Source: CAD feature listing. Evaluate the final solid. Frame: model axes, mm. A direction names the side the tool comes from. Round coordinates to 2 decimals unless told otherwise and drop trailing zeros. Loops run counter-clockwise (first coordinate to the right, second up) from the corner with the lowest first, then second, coordinate; pieces in that order, holes last.
Item 1: Section query D-D on y = 2.65. Give the number of separate pieces and of enclosed holes in the cut face, then the cut area to 3 significant figures.
Item 2: First-contact query: P1, Ø4, axis at x = 14, z = 0, coming from the +Y side; P2, Ø5, axis at x = 0, z = -14, coming from the +Y side; P3, Ø2, axis at x = 51.5, y = 1.5, coming from the -Z side; P4, Ø1.2, axis at x = 43, y = 2, coming from the +Z side. Flat tips, straight axial feed; report the tip coordinate or a pass-through.
Item 3: Section query B-B on z = -22.5. Return loops of the section in (x, y).
Item 4: Section query C-C on x = 25. Return loops of the section in (y, z).
Item 5: Pull-direction query (X, two-part tool) for faces 1 (the cylindrical face through (26.16, 1.97, 11.18)), 2 (the flat face through (-28.284, 2, 0)), 3 (the flat face through (41, 2, -15.91)); classes: released by +X, released by -X, zero draft, split by the parting line, or undercut.
Item 6: Access query for faces 4 (the flat face through (41, 2, 15.91)), 5 (the cylindrical face through (0.09, 1.97, 11.9)). Directions: +Z, -Z, +X, -X, +Y, -Y. A direction counts if a zero-diameter tool reaches every point of the face in a straight line with its end or side. Return the directions, or none.
Item 7: Ray query, L1, parallel to X at y = 1.8, z = 0; L2, parallel to Z at x = 59.5, y = 1.1; L3, parallel to Z at x = 50, y = 2.4. Return the intervals inside material, ascending.
Item 8: Section query A-A on x = 0. Return loops of the section in (y, z).
```python
from build123d import *

# Parameters (mm, degrees)
SKETCH_1_R          = 2.1
SKETCH_1_R_2        = 10.5
SKETCH_1_R_3        = 10
EXTRUDE_1_DEPTH     = 4
CHAMFER_1_SIZE      = 5
FILLET_1_R          = 10
SKETCH_2_R          = 2.1
CUT_EXTRUDE_1_DEPTH = 10
EXTRUDE_START       = -3
SKETCH_3_R          = 1.6
EXTRUDE_2_DEPTH     = 3
FILLET_2_R          = 3
FILLET_3_R          = 11
SKETCH_4_R          = 1.6
EXTRUDE_3_DEPTH     = 3
FILLET_4_R          = 10
CHAMFER_2_SIZE      = 2
CHAMFER_2_SIZE2     = 1.851556395
FILLET_5_R          = 10
CUT_EXTRUDE_START   = -10
CUT_EXTRUDE_2_DEPTH = 10
CUT_EXTRUDE_3_DEPTH = 10
CHAMFER_3_SIZE      = 5


with BuildPart() as part:
    # 草图1 → 凸台-拉伸1 (new body)
    with BuildSketch(Plane(origin=(0, 0, 0), x_dir=(1, 0, 0), z_dir=(0, 1, 0))):
        Polygon((0, 31.819805153), (-31.819805153, 0), (0, -31.819805153), (15.909902577, -15.909902577), (67.5, -15.909902577), (67.5, -22.5), (112.5, -22.5), (112.5, 22.5), (67.5, 22.5), (67.5, 15.909902577), (15.909902577, 15.909902577), align=None)
        with Locations(Location((0, 14, 0), (0, 0, 270))):
            Circle(SKETCH_1_R, mode=Mode.SUBTRACT)
        with Locations(Location((14, 0, 0), (0, 0, 270))):
            Circle(SKETCH_1_R, mode=Mode.SUBTRACT)
        with Locations(Location((0, -14, 0), (0, 0, 270))):
            Circle(SKETCH_1_R, mode=Mode.SUBTRACT)
        with Locations(Location((-14, 0, 0), (0, 0, 270))):
            Circle(SKETCH_1_R, mode=Mode.SUBTRACT)
        with Locations(Location((90, 0, 0), (0, 0, 270))):
            Circle(SKETCH_1_R_2, mode=Mode.SUBTRACT)
        with Locations(Location((0, 22.5, 0), (0, 0, 270))):
            Circle(SKETCH_1_R, mode=Mode.SUBTRACT)
        with Locations(Location((0, -22.5, 0), (0, 0, 270))):
            Circle(SKETCH_1_R, mode=Mode.SUBTRACT)
        with Locations(Location((0, 0, 0), (0, 0, 270))):
            Circle(SKETCH_1_R_3, mode=Mode.SUBTRACT)
        with Locations(Location((-22.5, 0, 0), (0, 0, 270))):
            Circle(SKETCH_1_R, mode=Mode.SUBTRACT)
    extrude(amount=EXTRUDE_1_DEPTH)

    # 倒角1
    chamfer_1_edges = [part.edges().sort_by_distance(p)[0] for p in [
        (112.5, 2, -22.5),
        (112.5, 2, 22.5),
        (0, 2, 31.819805153),
        (-31.819805153, 2, 0),
        (0, 2, -31.819805153),
    ]]
    chamfer(chamfer_1_edges, length=CHAMFER_1_SIZE)

    # 圆角1
    # the kernel refuses this fillet: 10 mm, written as the material it adds along each edge
    with BuildSketch(Plane(origin=(15.909902577, 0, -15.909902577), x_dir=(-0.707106781186552, 0, -0.707106781186543), z_dir=(0, 1, 0))) as fillet_1_piece_1:
        with BuildLine():
            CenterArc((FILLET_1_R * 0.414213562373, -FILLET_1_R), FILLET_1_R, 90, 45)
            Line((-FILLET_1_R * 0.292893218813, -FILLET_1_R * 0.292893218813), (-FILLET_1_R * 0.307035354437, -FILLET_1_R * 0.27875108319))
            Line((-FILLET_1_R * 0.307035354437, -FILLET_1_R * 0.27875108319), (-FILLET_1_R * 0.00828427124746, FILLET_1_R * 0.02))
            Line((-FILLET_1_R * 0.00828427124746, FILLET_1_R * 0.02), (FILLET_1_R * 0.414213562373, FILLET_1_R * 0.02))
            Line((FILLET_1_R * 0.414213562373, FILLET_1_R * 0.02), (FILLET_1_R * 0.414213562373, 0))
        make_face()
    extrude(amount=4)
    with BuildSketch(Plane(origin=(15.909902577, 0, 15.909902577), x_dir=(-0.7071067811865422, 0, 0.707106781186553), z_dir=(0, 1, 0))) as fillet_1_piece_2:
        with BuildLine():
            CenterArc((FILLET_1_R * 0.414213562373, FILLET_1_R), FILLET_1_R, 225, 45)
            Line((-FILLET_1_R * 0.292893218813, FILLET_1_R * 0.292893218813), (-FILLET_1_R * 0.307035354437, FILLET_1_R * 0.27875108319))
            Line((-FILLET_1_R * 0.307035354437, FILLET_1_R * 0.27875108319), (-FILLET_1_R * 0.00828427124746, -FILLET_1_R * 0.02))
            Line((-FILLET_1_R * 0.00828427124746, -FILLET_1_R * 0.02), (FILLET_1_R * 0.414213562373, -FILLET_1_R * 0.02))
            Line((FILLET_1_R * 0.414213562373, -FILLET_1_R * 0.02), (FILLET_1_R * 0.414213562373, 0))
        make_face()
    extrude(amount=4)
    with BuildSketch(Plane(origin=(67.5, 0, 15.909902577), x_dir=(-1, 0, 0), z_dir=(0, 1, 0))) as fillet_1_piece_3:
        with BuildLine():
            CenterArc((9.400668296, 10), FILLET_1_R, 199.937217397, 70.062782603)
            Line((0, 6.590097423), (-0.188013366, 6.521899372))
            ThreePointArc((-0.188013366, 6.521899372), (-0.2, 3.295048712), (-0.2, 0))
            Line((-0.2, 0), (0, -0.2))
            Line((0, -0.2), (9.400668296, -0.2))
            Line((9.400668296, -0.2), (9.400668296, 0))
        make_face()
    extrude(amount=4)
    with BuildSketch(Plane(origin=(67.5, 0, -15.909902577), x_dir=(-1, 0, 0), z_dir=(0, 1, 0))) as fillet_1_piece_4:
        with BuildLine():
            CenterArc((9.400668296, -10), FILLET_1_R, 90, 70.062782603)
            Line((0, -6.590097423), (-0.188013366, -6.521899372))
            ThreePointArc((-0.188013366, -6.521899372), (-0.2, -3.295048712), (-0.2, 0))
            Line((-0.2, 0), (0, 0.2))
            Line((0, 0.2), (9.400668296, 0.2))
            Line((9.400668296, 0.2), (9.400668296, 0))
        make_face()
    extrude(amount=4)

    # 草图2 → 切除-拉伸1 (cut)
    with BuildSketch(Plane.XZ):
        with Locations(Location((106.464466094, 16.464466094, 0), (0, 0, 270))):
            Circle(SKETCH_2_R)
        with Locations(Location((106.464466094, -16.464466094, 0), (0, 0, 270))):
            Circle(SKETCH_2_R)
        with Locations(Location((73.535533906, -16.464466094, 0), (0, 0, 90))):
            Circle(SKETCH_2_R)
        with Locations(Location((73.535533906, 16.464466094, 0), (0, 0, 90))):
            Circle(SKETCH_2_R)
        with Locations(Location((24.075684952, 10.909902577, 0), (0, 0, 270))):
            Circle(SKETCH_2_R)
        with Locations(Location((59.075684952, 10.909902577, 0), (0, 0, 270))):
            Circle(SKETCH_2_R)
        with Locations(Location((59.075684952, -10.909902577, 0), (0, 0, 90))):
            Circle(SKETCH_2_R)
        with Locations(Location((24.075684952, -10.909902577, 0), (0, 0, 90))):
            Circle(SKETCH_2_R)
    extrude(amount=-CUT_EXTRUDE_1_DEPTH, mode=Mode.SUBTRACT)

    # 草图3 → 凸台-拉伸2 (add)
    with BuildSketch(Plane(origin=(0, 4, 0), x_dir=(1, 0, 0), z_dir=(0, 1, 0)).offset(EXTRUDE_START)):
        with BuildLine():
            Line((3.535533906, 28.284271247), (40.057636417, 81.344203773))
            ThreePointArc((40.057636417, 81.344203773), (45.94930127, 83.86671265), (50.75784592, 79.629654221))
            Line((50.75784592, 79.629654221), (67.5, 22.5))
            ThreePointArc((67.5, 22.5), (63.839583189, 17.721525883), (58.099331704, 15.909902577))
            Line((58.099331704, 15.909902577), (20.0520382, 15.909902577))
            ThreePointArc((20.0520382, 15.909902577), (16.225203877, 16.671107252), (12.980970389, 18.838834765))
            Line((12.980970389, 18.838834765), (3.535533906, 28.284271247))
        make_face()
        with Locations(Location((45, 77.942286341, 0), (0, 0, 270))):
            Circle(SKETCH_3_R, mode=Mode.SUBTRACT)
        Polygon((16.491758356, 29.470182421), (43.526560522, 68.746803428), (56.080145943, 25.909902577), (20.0520382, 25.909902577), align=None, mode=Mode.SUBTRACT)
    extrude(amount=EXTRUDE_2_DEPTH)

    # 圆角2
    fillet_2_edges = [part.edges().sort_by_distance(p)[0] for p in [
        (16.491758356, 2.5, -29.470182421),
        (43.526560522, 2.5, -68.746803428),
        (56.080145943, 2.5, -25.909902577),
        (20.0520382, 2.5, -25.909902577),
    ]]
    fillet(fillet_2_edges, radius=FILLET_2_R)

    # 圆角3
    fillet_3_edges = [part.edges().sort_by_distance(p)[0] for p in [
        (3.535533906, 2.5, -28.284271247),
        (67.5, 2.5, -22.5),
    ]]
    fillet(fillet_3_edges, radius=FILLET_3_R)

    # 草图4 → 凸台-拉伸3 (add)
    with BuildSketch(Plane(origin=(0, 4, 0), x_dir=(1, 0, 0), z_dir=(0, 1, 0)).offset(EXTRUDE_START)):
        with BuildLine():
            Line((45.94930127, 83.86671265), (81.347717681, 83.86671265))
            Line((81.347717681, 83.86671265), (107.5, 22.5))
            Line((107.5, 22.5), (97.716806526, 22.5))
            Line((97.716806526, 22.5), (75.4, 74.86671265))
            Line((75.4, 74.86671265), (52.153651701, 74.86671265))
            Line((52.153651701, 74.86671265), (50.75784592, 79.629654221))
            ThreePointArc((50.75784592, 79.629654221), (48.966689034, 82.443994695), (45.94930127, 83.86671265))
        make_face()
        with Locations(Location((78, 77.942286341, 0), (0, 0, 270))):
            Circle(SKETCH_4_R, mode=Mode.SUBTRACT)
    extrude(amount=EXTRUDE_3_DEPTH)

    # 圆角4
    fillet_4_edges = [part.edges().sort_by_distance(p)[0] for p in [
        (97.716806526, 2.5, -22.5),
        (75.4, 2.5, -74.86671265),
        (52.153651701, 2.5, -74.86671265),
    ]]
    fillet(fillet_4_edges, radius=FILLET_4_R)

    # 倒角2
    chamfer_2_edges = [part.edges().sort_by_distance(p)[0] for p in [
        (81.347717681, 2.5, -83.86671265),
    ]]
    chamfer_2_side = [part.faces().sort_by_distance(p)[0] for p in [
        (63.648509476, 2.5, -83.86671265),
    ]]
    chamfer(chamfer_2_edges, length=CHAMFER_2_SIZE, length2=CHAMFER_2_SIZE2, reference=chamfer_2_side[0])

    # 圆角5
    fillet_5_edges = [part.edges().sort_by_distance(p)[0] for p in [
        (107.5, 2.5, -22.5),
    ]]
    fillet(fillet_5_edges, radius=FILLET_5_R)

    # 草图5 → 切除-拉伸2 (cut)
    with BuildSketch(Plane(origin=(0, 4, 0), x_dir=(1, 0, 0), z_dir=(0, 1, 0)).offset(CUT_EXTRUDE_START)):
        with BuildLine():
            Line((67.5, -22.5), (67.5, -34.552858439))
            Line((67.5, -34.552858439), (139.474887753, -46.263885721))
            Line((139.474887753, -46.263885721), (130.519396302, 71.535271055))
            Line((130.519396302, 71.535271055), (50.264415224, 107.357236858))
            Line((50.264415224, 107.357236858), (-15.814227001, 52.524784707))
            Line((-15.814227001, 52.524784707), (-3.535533906, 28.284271247))
            Line((-3.535533906, 28.284271247), (3.535533906, 28.284271247))
            Line((3.535533906, 28.284271247), (12.980970389, 18.838834765))
            ThreePointArc((12.980970389, 18.838834765), (16.225203877, 16.671107252), (20.0520382, 15.909902577))
            Line((20.0520382, 15.909902577), (58.099331704, 15.909902577))
            ThreePointArc((58.099331704, 15.909902577), (63.839583189, 17.721525883), (67.5, 22.5))
            Line((67.5, 22.5), (67.5, -22.5))
        make_face()
    extrude(amount=CUT_EXTRUDE_2_DEPTH, mode=Mode.SUBTRACT)

    # 草图6 → 切除-拉伸3 (cut)
    with BuildSketch(Plane(origin=(0, 4, 0), x_dir=(1, 0, 0), z_dir=(0, 1, 0))):
        Polygon((58.099331704, 15.909902577), (80.044473587, 15.909902577), (76.388599313, 31.9888999), (52.293064323, 28.831553936), align=None)
        Polygon((58.099331704, -15.909902577), (78.21653645, -15.909902577), (69.071902646, -30.327138866), (59.799179703, -28.451958172), align=None)
    extrude(amount=-CUT_EXTRUDE_3_DEPTH, mode=Mode.SUBTRACT)

    # 倒角3
    chamfer_3_edges = [part.edges().sort_by_distance(p)[0] for p in [
        (67.5, 2, -15.909902577),
        (67.5, 2, 15.909902577),
    ]]
    chamfer(chamfer_3_edges, length=CHAMFER_3_SIZE)


solid = part.part
```
Data:
1. separate pieces: 1
1. enclosed holes: 12
1. area: 2,890 mm2
2. P1: passes through
2. P2: stops at y = 4
2. P3: stops at z = -15.91
2. P4: stops at z = 15.91
3. outline: (-9.32, 0) - (-2.1, 0) - (-2.1, 4) - (-9.32, 4) - close; (2.1, 0) - (9.32, 0) - (9.32, 4) - (2.1, 4) - close
4. outline: (0, -15.91) - (4, -15.91) - (4, -12.8) - (0, -12.8) - close; (0, -9.02) - (4, -9.02) - (4, 9.02) - (0, 9.02) - close; (0, 12.8) - (4, 12.8) - (4, 15.91) - (0, 15.91) - close
5. face 1: undercut
5. face 2: released by -X
5. face 3: zero draft
6. face 4: +Z, +X, +Y, -Y
6. face 5: +Y, -Y
7. L1: x = -28.28 to -24.6, -20.4 to -16.1, -11.9 to -10, 10 to 11.9, 16.1 to 67.5
7. L2: z = -15.91 to -12.97, -8.85 to 8.85, 12.97 to 15.91
7. L3: z = -15.91 to 15.91
8. outline: (0, -28.28) - (4, -28.28) - (4, -24.6) - (0, -24.6) - close; (0, -20.4) - (4, -20.4) - (4, -16.1) - (0, -16.1) - close; (0, -11.9) - (4, -11.9) - (4, -10) - (0, -10) - close; (0, 10) - (4, 10) - (4, 11.9) - (0, 11.9) - close; (0, 16.1) - (4, 16.1) - (4, 20.4) - (0, 20.4) - close; (0, 24.6) - (4, 24.6) - (4, 28.28) - (0, 28.28) - close
